from build123d import *

# Parameters (mm, degrees)
SKETCH1_R           = 7.5
BOSS_EXTRUDE1_DEPTH = 4
SKETCH2_R           = 6.5
CUT_EXTRUDE1_DEPTH  = 3
FILLET1_R           = 1
FILLET2_R           = 1


with BuildPart() as part:
    # Sketch1 → Boss-Extrude1 (new body)
    with BuildSketch(Plane(origin=(0, 0, 0), x_dir=(1, 0, 0), z_dir=(0, 1, 0))):
        with Locations(Location((0, 0, 0), (0, 0, 270))):
            Circle(SKETCH1_R)
    extrude(amount=BOSS_EXTRUDE1_DEPTH)

    # Sketch2 → Cut-Extrude1 (cut)
    with BuildSketch(Plane(origin=(0, 4, 0), x_dir=(1, 0, 0), z_dir=(0, 1, 0))):
        with Locations(Location((0, 0, 0), (0, 0, 270))):
            Circle(SKETCH2_R)
    extrude(amount=-CUT_EXTRUDE1_DEPTH, mode=Mode.SUBTRACT)

    # Fillet1
    fillet1_edges = [part.edges().sort_by_distance(p)[0] for p in [
        (0, 4, -7.5),
    ]]
    fillet(fillet1_edges, radius=FILLET1_R - 0.0001)  # a hair under: the kernel refuses the full size

    # Fillet2
    fillet2_edges = [part.edges().sort_by_distance(p)[0] for p in [
        (0, 0, -7.5),
    ]]
    fillet(fillet2_edges, radius=FILLET2_R)


solid = part.part
Read the model definition and answer for the solid it produces. Units are mm, in the model's axes. Coordinates: 2 decimals unless noted, no trailing zeros. Loops run counter-clockwise (first coordinate to the right, second up) from the corner with the lowest first, then second, coordinate; pieces in that order, holes last.
Q1. Consider probe 1 along X at (y, z) = (2, 0); probe 2 along Y at (x, z) = (-3, 1.75); probe 3 along X at (y, z) = (3.5, -1.5). Determine where each line is inside the solid, lowest interval first.
Q2. The part is cut by section B-B on y = 1.3. Write down the section's boundary in (x, z).
Q3. The mould has two halves that part along Z. Classify faces 1 (the face through (0, 1, 0)), 2 (the face through (0.33, 1.986, -7.493)), 3 (the face through (0, 0, 0)): +Z half, -Z half, draft (parallel to the pull), parting line (faces both ways), or undercut.
Q4. The part is cut by section D-D on y = 0.3. Write down the section's boundary in (x, z).
Q5. This flat-tipped pin is pushed along its axis until it touches: pin 1 Ø4 at (x, z) = (2, -2) entering from +Y. Where does it stop, or does it pass through?
Results below:
1. probe 1: x = -7.5 to -6.5, 6.5 to 7.5
1. probe 2: y = 0 to 1
1. probe 3: x = -7.21 to -6.32, 6.32 to 7.21
2. outline: circle Ø15 at (0, 0); hole circle Ø13 at (0, 0)
3. face 1: undercut
3. face 2: parting line
3. face 3: draft
4. outline: circle Ø14.43 at (0, 0)
5. pin 1: stops at y = 1
